Here's how the part is built. I have some questions about the finished solid (model axes, mm). A direction names the side the tool comes from. Round coordinates to 2 decimals unless told otherwise and drop trailing zeros. Loops run counter-clockwise (first coordinate to the right, second up) from the corner with the lowest first, then second, coordinate; pieces in that order, holes last. Notation, with made-up numbers: M 4,29.5 L 56,29.5 A11 cw 56,40.5 Z; hole C -2,12 d5. An arc over 180 degrees is marked long. Write each question's results on one line, items separated by ' | '. Start each with the question number.
```python
from build123d import *

# Parameters (mm, degrees)
ESBO_O1_R                = 2
RESSALTO_EXTRUS_O1_DEPTH = 19
CORTE_EXTRUS_O1_DEPTH    = 18
ESBO_O3_R                = 2.5
RESSALTO_EXTRUS_O2_DEPTH = 7


with BuildPart() as part:
    # Esboço1 → Ressalto-extrusão1 (new body)
    with BuildSketch(Plane.XY):
        with BuildLine():
            Line((17.5, 3.5), (13.555441712, 3.5))
            ThreePointArc((13.555441712, 3.5), (0, 14), (-13.555441712, 3.5))
            Line((-13.555441712, 3.5), (-17.5, 3.5))
            ThreePointArc((-17.5, 3.5), (-21, 0), (-17.5, -3.5))
            Line((-17.5, -3.5), (-13.555441712, -3.5))
            ThreePointArc((-13.555441712, -3.5), (-11.320120282, -8.237407166), (-7.5, -11.821590418))
            Line((-7.5, -11.821590418), (-7.5, -14))
            Line((-7.5, -14), (-7.5, -17))
            Line((-7.5, -17), (7.5, -17))
            Line((7.5, -17), (7.5, -14))
            Line((7.5, -14), (7.5, -11.821590418))
            ThreePointArc((7.5, -11.821590418), (11.320120282, -8.237407166), (13.555441712, -3.5))
            Line((13.555441712, -3.5), (17.5, -3.5))
            ThreePointArc((17.5, -3.5), (21, 0), (17.5, 3.5))
        make_face()
        with Locations((17.5, 0)):
            Circle(ESBO_O1_R, mode=Mode.SUBTRACT)
        with Locations((-17.5, 0)):
            Circle(ESBO_O1_R, mode=Mode.SUBTRACT)
    extrude(amount=RESSALTO_EXTRUS_O1_DEPTH)

    # Esboço2 → Corte-extrusão1 (cut)
    with BuildSketch(Plane(origin=(0, 0, 0), x_dir=(-1, 0, 0), z_dir=(0, 0, -1))):
        with BuildLine():
            Line((13.555441712, 3.5), (23.80699558, 3.5))
            Line((23.80699558, 3.5), (23.80699558, -3.5))
            Line((23.80699558, -3.5), (13.555441712, -3.5))
            ThreePointArc((13.555441712, -3.5), (14, 0), (13.555441712, 3.5))
        make_face()
        with BuildLine():
            Line((-13.555441712, 3.5), (-24.760546325, 3.5))
            Line((-24.760546325, 3.5), (-24.760546325, -3.5))
            Line((-24.760546325, -3.5), (-13.555441712, -3.5))
            ThreePointArc((-13.555441712, -3.5), (-14, 0), (-13.555441712, 3.5))
        make_face()
    extrude(amount=-CORTE_EXTRUS_O1_DEPTH, mode=Mode.SUBTRACT)

    # Esboço3 → Ressalto-extrusão2 (add)
    with BuildSketch(Plane.XY.offset(19)):
        with Locations((0, 6.5)):
            Circle(ESBO_O3_R)
    extrude(amount=RESSALTO_EXTRUS_O2_DEPTH)


solid = part.part
```
Item 1: I'm going to push flat-ended pins straight in: pin 1 (0.5 mm diameter, centred on x = -14.5, z = 18.5, fed in from -Y); pin 2 (6 mm diameter, centred on x = 5, z = 20.5, fed in from +Y); pin 3 (1.1 mm diameter, centred on x = -15.5, z = 18.5, fed in from +Y); pin 4 (2 mm diameter, centred on x = 15, y = -5, fed in from +Z). Where does each tip first touch, or does it pass through?
Item 2: If we mould it in two halves opening along X, with no side actions, what happens to faces 1 (the face through (-19.1, -1.2, 18.5)), 2 (the face through (7.5, -14, 9)), 3 (the face through (-7.5, -14, 9))? For each: released by +X, released by -X, zero draft, split by the parting line, or undercut.
Item 3: If we section it at D-D on y = -4: Please give me the cut outline in (x, z), and give its area (3 significant figures).
Item 4: If we section it at B-B on x = 0: Please give me the cut outline in (y, z), and give its area (3 significant figures).
Item 5: If we section it at A-A on x = 17: Please give me the cut outline in (y, z).
Item 6: If we section it at C-C on z = 9: Please give me the cut outline in (x, y).
Item 7: I need wall thicknesses on L1, parallel to X at y = 0, z = 18.5; L2, parallel to Y at x = -17.5, z = 18.45; L3, parallel to Z at x = 10.5, y = -7. Which ranges of each line are inside material? Lowest first, please.
Item 8: Which directions (+Z, -Z, +X, -X, +Y, -Y) give clear straight access to the entire face, cutting with the end or side of a thin tool? Please do faces 4 (the face through (15.6, 3.5, 18.5)), 5 (the face through (15.5, -3.5, 18.5)), 6 (the face through (-15.5, 3.5, 18.5)).
Numbers:
1) pin 1: y = -3.5 | pin 2: y = 13.79 | pin 3: y = 3.5 | pin 4: through
2) face 1: undercut | face 2: released by +X | face 3: released by -X
3) outline: M -13.42,0 L 13.42,0 L 13.42,19 L -13.42,19 Z | area: 510 mm²
4) outline: M -17,0 L 14,0 L 14,19 L 9,19 L 9,26 L 4,26 L 4,19 L -17,19 Z | area: 624 mm²
5) outline: M -3.5,18 L -1.94,18 L -1.94,19 L -3.5,19 Z; M 1.94,18 L 3.5,18 L 3.5,19 L 1.94,19 Z
6) outline: M -7.5,-17 L 7.5,-17 L 7.5,-11.82 A14 ccw long -7.5,-11.82 Z
7) L1: -21 to -19.5, -15.5 to 15.5, 19.5 to 21 | L2: -3.5 to -2, 2 to 3.5 | L3: 0 to 19
8) face 4: +Z, -Z, +X, +Y | face 5: +Z, -Z, +X, -Y | face 6: +Z, -Z, -X, +Y
